Verification items for the finished model (mm, model axes). Round coordinates to 2 decimals unless told otherwise and drop trailing zeros. Loops run counter-clockwise (first coordinate to the right, second up) from the corner with the lowest first, then second, coordinate; pieces in that order, holes last. Notation, with made-up numbers: (82.25, 70.5) - (115.25, 70.5) arc R9 cw to (115.25, 85.5) - close; hole circle Ø8 at (74.5, 20.5). An arc over 180 degrees is marked (long way). Use CSV: the item, a comma, the result in double quotes.
```python
from build123d import *

# Parameters (mm, degrees)
F0_R     = 1.575
F1_DEPTH = 3
F2_R     = 5
F3_R     = 12
F4_W     = 3.2
F4_H     = 4
F4_W_2   = 4
F4_H_2   = 3.2
F5_DEPTH = 2
F6_R     = 0.5
F7_SIZE  = 0.25


with BuildPart() as f1:
    # F0 (on Front) → F1 (new body)
    with BuildSketch(Plane.XZ):
        Polygon((7.25, 7.25), (7.25, 45), (-7.25, 45), (-7.25, -7.25), (45, -7.25), (45, 7.25), align=None)
        with Locations((22.5, 0)):
            Circle(F0_R, mode=Mode.SUBTRACT)
        with Locations((37.5, 0)):
            Circle(F0_R, mode=Mode.SUBTRACT)
        with Locations((0, 22.5)):
            Circle(F0_R, mode=Mode.SUBTRACT)
        with Locations((0, 37.5)):
            Circle(F0_R, mode=Mode.SUBTRACT)
    extrude(amount=F1_DEPTH)

    # F2
    f2_edges = [f1.edges().sort_by_distance(p)[0] for p in [
        (-7.25, -1.5, 45),
        (7.25, -1.5, 45),
        (45, -1.5, 7.25),
        (45, -1.5, -7.25),
    ]]
    fillet(f2_edges, radius=F2_R)

    # F3
    f3_edges = [f1.edges().sort_by_distance(p)[0] for p in [
        (7.25, -1.5, 7.25),
        (-7.25, -1.5, -7.25),
    ]]
    fillet(f3_edges, radius=F3_R)

    # F4 (on face) → F5 (join)
    with BuildSketch(Plane.XZ.offset(3)):
        with Locations((0, 30)):
            Rectangle(F4_W, F4_H)
        with Locations((30, 0)):
            Rectangle(F4_W_2, F4_H_2)
    extrude(amount=F5_DEPTH)

    # F6
    f6_edges = [f1.edges().sort_by_distance(p)[0] for p in [
        (28, -4, -1.6),
        (32, -4, -1.6),
        (32, -4, 1.6),
        (28, -4, 1.6),
        (-1.6, -4, 28),
        (-1.6, -4, 32),
        (1.6, -4, 28),
        (1.6, -4, 32),
    ]]
    fillet(f6_edges, radius=F6_R)

    # F7
    f7_edges = [f1.edges().sort_by_distance(p)[0] for p in [
        (7.25, 0, 29.625),
        (10.764719, 0, 10.764719),
        (5.785534, 0, 43.535534),
        (29.625, 0, 7.25),
        (0, 0, 45),
        (43.535534, 0, 5.785534),
        (-5.785534, 0, 43.535534),
        (45, 0, 0),
        (-7.25, 0, 22.375),
        (43.535534, 0, -5.785534),
        (-3.735281, 0, -3.735281),
        (22.375, 0, -7.25),
        (20.925, 0, 0),
        (35.925, 0, 0),
        (-1.575, 0, 22.5),
        (-1.575, 0, 37.5),
    ]]
    chamfer(f7_edges, length=F7_SIZE)


solid = f1.part
```
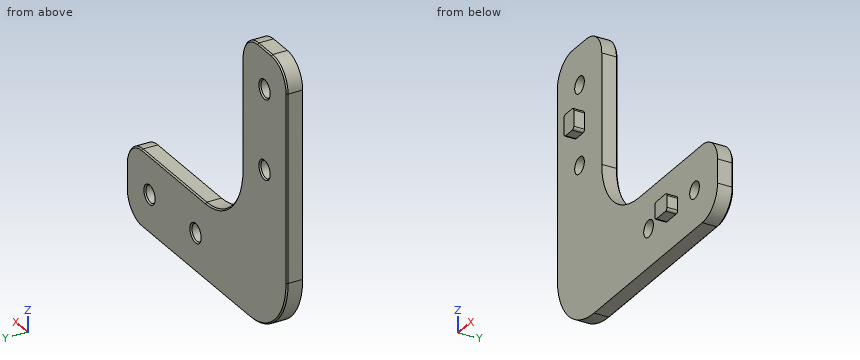
1) Cross-section at A-A, the plane z = 37.5. Record the cut outline in (x, y) (3 decimals), then the cut area to 3 significant figures.
Returned:
outline,"(-7.25, -3) - (-1.575, -3) - (-1.575, -0.25) - (-1.825, 0) - (-7, 0) - (-7.25, -0.25) - close; (1.575, -3) - (7.25, -3) - (7.25, -0.25) - (7, 0) - (1.825, 0) - (1.575, -0.25) - close"
area,"33.9 mm²"
2) Cross-section at C-C, the plane x = 22.5. Record the cut outline in (y, z) (3 decimals).
Returned:
outline,"(-3, -7.25) - (-0.25, -7.25) - (0, -7) - (0, -1.825) - (-0.25, -1.575) - (-3, -1.575) - close; (-3, 1.575) - (-0.25, 1.575) - (0, 1.825) - (0, 7) - (-0.25, 7.25) - (-3, 7.25) - close"
3) Cross-section at D-D, the plane x = 0. Count the separate pieces of the cut face and the enclosed holes in it, then the cut area to 3 significant figures.
Returned:
separate pieces,"3"
enclosed holes,"0"
area,"143 mm²"
4) Thickness scan on probe 1 along Z at (x, y) = (37.5, -1.9) (3 decimals); probe 2 along Z at (x, y) = (0, -1.95) (3 decimals). Record the ranges inside material, lowest first. Write a range as [from, to].
Returned:
probe 1,"z = [-7.25, -1.575], [1.575, 7.25]"
probe 2,"z = [-6.27, 20.925], [24.075, 35.925], [39.075, 45]"
5) Cross-section at B-B, the plane y = -2.1. Record the cut outline in (x, z) (3 decimals), then the cut area to 3 significant figures.
Returned:
outline,"(-7.25, 4.75) arc R12 ccw to (4.75, -7.25) - (40, -7.25) arc R5 ccw to (45, -2.25) - (45, 2.25) arc R5 ccw to (40, 7.25) - (19.25, 7.25) arc R12 cw to (7.25, 19.25) - (7.25, 40) arc R5 ccw to (2.25, 45) - (-2.25, 45) arc R5 ccw to (-7.25, 40) - close; hole circle Ø3.15 at (0, 22.5); hole circle Ø3.15 at (0, 37.5); hole circle Ø3.15 at (22.5, 0); hole circle Ø3.15 at (37.5, 0)"
area,"1,250 mm²"
6) Gauge pin test, flat ends, axial feed: pin 1 Ø1.6 at (y, z) = (-4.5, -0.5) entering from +X; pin 2 Ø1 at (x, y) = (0, -4) entering from +Z; pin 3 Ø1.6 at (y, z) = (-4, 30) entering from -X; pin 4 Ø1.9 at (x, z) = (22.5, 0) entering from +Y. Record the tip position at first contact, or that the pin passes through.
Returned:
pin 1,"stops at x = 32"
pin 2,"stops at z = 32"
pin 3,"stops at x = -1.6"
pin 4,"passes through"
